Can you work these out from the drawing? Everything is in mm from the part's minimum corner. A direction names the side the tool comes from. Coordinates: 2 decimals unless noted, no trailing zeros. Loops run counter-clockwise (first coordinate to the right, second up) from the corner with the lowest first, then second, coordinate; pieces in that order, holes last.
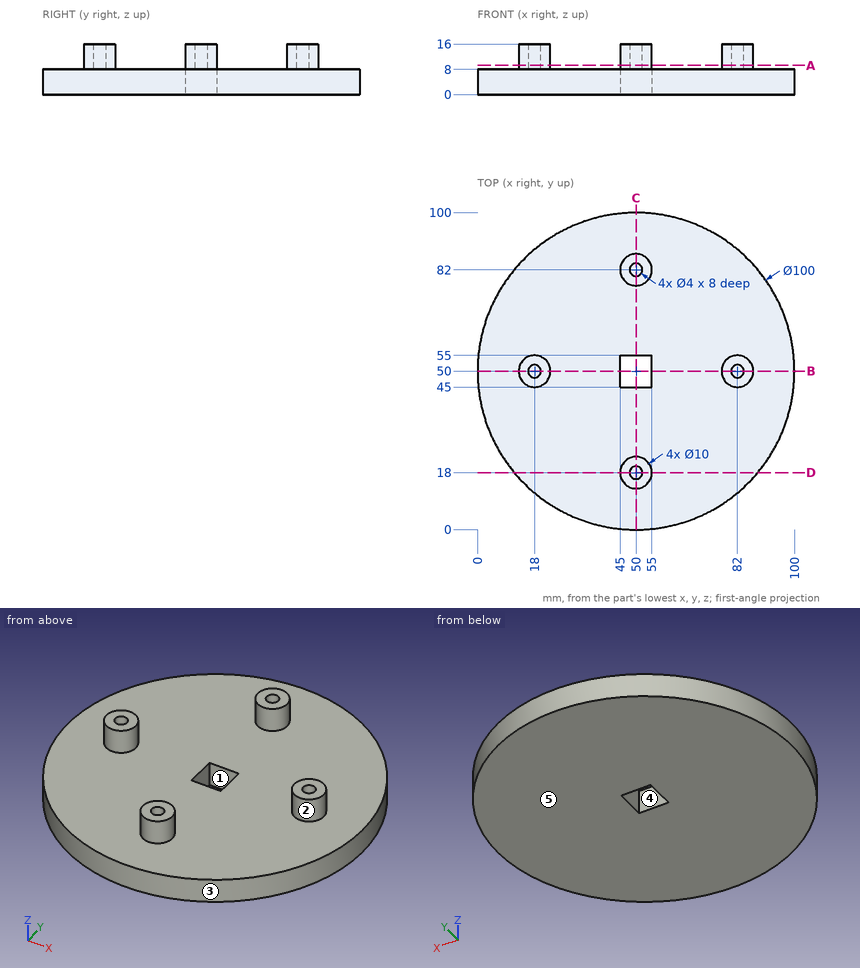
1) Will these pins go through, and if not, where does the flat tip stop? pin 1 (3 mm diameter, centred on y = 33.5, z = 5.5, fed in from -X); pin 2 (9 mm diameter, centred on x = 48, z = 5, fed in from -Y); pin 3 (6 mm diameter, centred on y = 27, z = 3, fed in from +X).
2) Imagine slicing it at B-B on y = 50. List the corners of the cut face in (x, z) for me, plus the area to 3 significant figures.
3) Imagine slicing it at A-A on z = 9.25. List the corners of the cut face in (x, y) for me, plus the area to 3 significant figures.
4) If I drill on L1, parallel to Y at x = 18, z = 12.5; L2, parallel to Y at x = 50, z = 10; L3, parallel to Z at x = 28, y = 73, over which ranges is the centre line in solid material (lowest first)?
5) For the marked faces 1 and 2, which set-ups out of +Z, -Z, +X, -X, +Y, -Y let a thin tool reach every point of the face, with its end or its side?
6) Imagine slicing it at D-D on y = 18. List the corners of the cut face in (x, z) for me.
7) We'd pull the mould along Y, two halves only. Please class the marked faces 3, 4 and 5: released by +Y, released by -Y, zero draft, split by the parting line, or undercut.
Solved:
1. pin 1: stops at x = 2.3
1. pin 2: stops at y = 0
1. pin 3: stops at x = 95.83
2. outline: (0, 0) - (45, 0) - (45, 8) - (23, 8) - (23, 16) - (20, 16) - (20, 8) - (16, 8) - (16, 16) - (13, 16) - (13, 8) - (0, 8) - close; (55, 0) - (100, 0) - (100, 8) - (87, 8) - (87, 16) - (84, 16) - (84, 8) - (80, 8) - (80, 16) - (77, 16) - (77, 8) - (55, 8) - close
2. area: 816 mm2
3. outline: circle Ø10 at (18, 50); circle Ø10 at (50, 18); circle Ø10 at (50, 82); circle Ø10 at (82, 50); hole circle Ø4 at (18, 50); hole circle Ø4 at (50, 18); hole circle Ø4 at (50, 82); hole circle Ø4 at (82, 50)
3. area: 264 mm2
4. L1: y = 45 to 48, 52 to 55
4. L2: y = 13 to 16, 20 to 23, 77 to 80, 84 to 87
4. L3: z = 0 to 8
5. face 1: +Z, -Z
5. face 2: +Z
6. outline: (11.58, 0) - (88.42, 0) - (88.42, 8) - (55, 8) - (55, 16) - (52, 16) - (52, 8) - (48, 8) - (48, 16) - (45, 16) - (45, 8) - (11.58, 8) - close
7. face 3: split by the parting line
7. face 4: undercut
7. face 5: zero draft
